from build123d import *

# Parameters (mm, degrees)
PAD_DEPTH       = 20
SKETCH001_R     = 1.5
POCKET_DEPTH    = 174.036499
POCKET001_DEPTH = 20.001
SKETCH003_W     = 13.051827
SKETCH003_H     = 6.909791
SKETCH003_W_2   = 4.990405
SKETCH003_H_2   = 12.476008
POCKET002_DEPTH = 3
SKETCH004_W     = 2
SKETCH004_H     = 5
PAD001_DEPTH    = 20
SKETCH005_W     = 66
SKETCH005_H     = 4
PAD002_DEPTH    = 8.5
SKETCH006_R     = 1
POCKET003_DEPTH = 13.501


with BuildPart() as part:
    # Sketch → Pad (new body)
    with BuildSketch(Plane.XZ):
        with BuildLine():
            Line((-35.5, 5), (35.5, 5))
            Line((35.5, 5), (35.5, 13.5))
            Line((35.5, 13.5), (38.5, 13.5))
            ThreePointArc((38.5, 9.5), (40.5, 11.5), (38.5, 13.5))
            Line((38.5, 9.5), (37.5, 9.5))
            Line((37.5, 9.5), (37.5, 0))
            Line((37.5, 0), (-37.5, 0))
            Line((-37.5, 0), (-37.5, 9.5))
            Line((-37.5, 9.5), (-38.5, 9.5))
            ThreePointArc((-38.5, 13.5), (-40.5, 11.5), (-38.5, 9.5))
            Line((-38.5, 13.5), (-35.5, 13.5))
            Line((-35.5, 13.5), (-35.5, 5))
        make_face()
    extrude(amount=PAD_DEPTH)

    # Sketch001 (on Face3 of Pad) → Pocket (cut, through all)
    with BuildSketch(Plane(origin=(0, 0, 5), x_dir=(-1, 0, 0), z_dir=(0, 0, 1))):
        with Locations((-13, 2.5)):
            Circle(SKETCH001_R)
        with Locations((-32, 2.5)):
            Circle(SKETCH001_R)
    pocket = extrude(amount=-POCKET_DEPTH, mode=Mode.SUBTRACT)

    # Mirrored: Pocket across Sketch001 V_Axis
    add(pocket.mirror(Plane(origin=(0, 0, 5), x_dir=(0, 0, 1), z_dir=(-1, 0, 0))), mode=Mode.SUBTRACT)

    # Sketch002 (on Face5 of Mirrored) → Pocket001 (cut, through all)
    with BuildSketch(Plane.XZ.offset(20)):
        with BuildLine():
            ThreePointArc((-8, 2), (-10, 0), (-8, -2))
            Line((-8, -2), (0, -2))
            ThreePointArc((0, -2), (2, 0), (0, 2))
            Line((-8, 2), (0, 2))
        make_face()
    extrude(amount=-POCKET001_DEPTH, mode=Mode.SUBTRACT)

    # Sketch003 → Pocket002 (cut)
    with BuildSketch(Plane(origin=(0, 0, 5), x_dir=(-1, 0, 0), z_dir=(0, 0, 1))):
        with Locations((-22.41574, 9.693542)):
            Rectangle(SKETCH003_W, SKETCH003_H)
        with Locations((-7.636473, 9.213694)):
            Rectangle(SKETCH003_W_2, SKETCH003_H_2)
    extrude(amount=-POCKET002_DEPTH, mode=Mode.SUBTRACT)

    # Sketch004 (on Face5 of Pocket002) → Pad001 (join)
    with BuildSketch(Plane.XZ.offset(20)):
        with Locations((-38.5, 2.5)):
            Rectangle(SKETCH004_W, SKETCH004_H)
        with Locations((38.5, 2.5)):
            Rectangle(SKETCH004_W, SKETCH004_H)
    extrude(amount=-PAD001_DEPTH)

    # Sketch005 (on Face7 of Pad001) → Pad002 (join)
    with BuildSketch(Plane(origin=(0, 0, 5), x_dir=(-1, 0, 0), z_dir=(0, 0, 1))):
        with Locations((0, 18)):
            Rectangle(SKETCH005_W, SKETCH005_H)
    extrude(amount=PAD002_DEPTH)

    # Sketch006 (on Face37 of Pad002) → Pocket003 (cut, through all)
    with BuildSketch(Plane(origin=(0, 0, 13.5), x_dir=(-1, 0, 0), z_dir=(0, 0, 1))):
        with Locations((0, 18)):
            Circle(SKETCH006_R)
        with Locations((28, 18)):
            Circle(SKETCH006_R)
        with Locations((-28, 18)):
            Circle(SKETCH006_R)
    extrude(amount=-POCKET003_DEPTH, mode=Mode.SUBTRACT)


solid = part.part
CAD build for the part. Positions are in the model's coordinates, mm. A direction names the side the tool comes from. Coordinates: 2 decimals unless noted, no trailing zeros. Write each loop counter-clockwise with the first axis right and the second up, starting at its lowest first coordinate (ties: lowest second). Pieces come first, ordered by that corner, then holes. Notation, with made-up numbers: M 69.5,-33 L 81.5,-33 A37 cw 81.5,4 Z; hole C 69,30 d8. An arc over 180 degrees is marked long. Return JSON: item names as keys, results as strings.
Item 1: Slice it at D-D, the plane y = -12.25. Write the cut outline in (x, z), and give its area (3 significant figures).
Findings below:
{"outline": "M -39.5,0 L -10,0 A2 cw -8,2 L 0,2 A2 cw 2,0 L 39.5,0 L 39.5,5 L 37.5,5 L 37.5,9.5 L 38.5,9.5 A2 ccw 38.5,13.5 L 35.5,13.5 L 35.5,5 L 28.94,5 L 28.94,2 L 15.89,2 L 15.89,5 L 10.13,5 L 10.13,2 L 5.14,2 L 5.14,5 L -35.5,5 L -35.5,13.5 L -38.5,13.5 A2 ccw -38.5,9.5 L -37.5,9.5 L -37.5,5 L -39.5,5 Z", "area": "373 mm2"}
Item 2: Drop flat-ended pins along their axis: pin 1 Ø2 at (y, z) = (-12, 7) entering from +X; pin 2 Ø1.5 at (y, z) = (-7, 3) entering from -X; pin 3 Ø2 at (x, y) = (20.5, -9) entering from +Z. Give the stop position or say it passes through.
Findings below:
{"pin 1": "stops at x = 37.5", "pin 2": "stops at x = -39.5", "pin 3": "stops at z = 2"}
Item 3: Slice it at A-A, the plane z = 11.5. Write the cut outline in (x, y).
Findings below:
{"outline": "M -40.5,-20 L -35.5,-20 L -35.5,0 L -40.5,0 Z; M -33,-20 L 33,-20 L 33,-16 L -33,-16 Z; M 35.5,-20 L 40.5,-20 L 40.5,0 L 35.5,0 Z; hole C -28,-18 d2; hole C 0,-18 d2; hole C 28,-18 d2"}
Item 4: Which spindle directions (+Z, -Z, +X, -X, +Y, -Y) get a long thin tool onto all of the face, cutting with end or side? Do faces 1 (the flat face through (0, -16, 9)), 2 (the flat face through (-37.5, -10, 7)), 3 (the flat face through (33, -18, 9)). Say none if no direction does.
Findings below:
{"face 1": "+Z, +Y", "face 2": "-X, +Y, -Y", "face 3": "+Z, +Y, -Y"}
Item 5: Slice it at C-C, the plane z = 4. State how many separate pieces and enclosed holes the cut face has, and give its area (3 significant figures).
Findings below:
{"separate pieces": "1", "enclosed holes": "9", "area": "1,390 mm2"}
Item 6: Probe line 1 (X direction, y = -2.5, z = 3.8); line 2 (Y direction, x = -13, z = 3.85); line 3 (Y direction, x = 0, z = 7.5). List the from-to ranges inside material, lowest first. Write a range as from..to.
Findings below:
{"line 1": "x = -39.5..-33.5, -30.5..-14.5, -11.5..11.5, 14.5..30.5, 33.5..39.5", "line 2": "y = -20..-4, -1..0", "line 3": "y = -20..-19, -17..-16"}
Item 7: Slice it at B-B, the plane x = 32. Write the cut outline in (y, z), and give its area (3 significant figures).
Findings below:
{"outline": "M -20,0 L -4,0 L -4,5 L -16,5 L -16,13.5 L -20,13.5 Z; M -1,0 L 0,0 L 0,5 L -1,5 Z", "area": "119 mm2"}
Item 8: Two-plate mould, pull along Z, no slides. Class faces 4 (the flat face through (-39, -10, 5)), 5 (the cylindrical face through (40.5, -9.9, 11.5)), 6 (the flat face through (23, -6.239, 4)), 7 (the cylindrical face through (1.43, -10.14, 1.4)): +Z half, -Z half, draft (parallel to the pull), parting line (faces both ways), or undercut.
Findings below:
{"face 4": "undercut", "face 5": "undercut", "face 6": "draft", "face 7": "-Z half"}
